For this review, take the finished solid that the model builds, in its own axes (mm). A direction names the side the tool comes from. Coordinates: 2 decimals unless noted, no trailing zeros. Write each loop counter-clockwise with the first axis right and the second up, starting at its lowest first coordinate (ties: lowest second). Pieces come first, ordered by that corner, then holes. Notation, with made-up numbers: (-31, 43) - (-5, 43) arc R16 cw to (-5, 56) - close; hole circle Ø1 at (43.5, -10). An arc over 180 degrees is marked (long way). Use one line per item in the form item = value. Start each with the question number.
1) We need section C-C (z = 0). Give the boundary of the cut face in (x, y), plus the area to 3 significant figures.
2) We need section B-B (y = 9.5). Give the boundary of the cut face in (x, z).
3) Mouldability with a two-part tool opening along Z and no side actions: class faces 3 (the flat face through (0, 0, 8)), 4 (the cylindrical face through (0.3, 11.6, -13.5)), 5 (the cylindrical face through (0.207, 11.661, 9.778)) as pulls with the +Z half, pulls with the -Z half, needs draft (parallel to the pull), parting line crosses it, or undercut.
4) Tool access review of faces 1 (the flat face through (0, 0.45, -15)), 2 (the cylindrical face through (0.3, 23.3, -3.6)): name each direction out of +Z, -Z, +X, -X, +Y, -Y from which nothing blocks a thin tool from reaching the whole face with its end or side.
5) Insertion check: P1, Ø1, axis at x = 0, z = -15.5, coming from the -Y side. The pin has a flat end and moves straight along its axis. Give the tip position at first contact, or say it passes through.
6) For L1, parallel to Z at x = -0.1, y = 21.5; L2, parallel to Y at x = -0.1, z = -7; L3, parallel to X at y = 25, z = 4, list the stretches that pass through material, from the lowest coordinate up. Write a range as from..to.
Autodesk Inventor part; units mm, degrees
ref_plane "YZ Plane" through (0, 0, 0) normal (1, 0, 0) x (0, 1, 0)
ref_plane "XZ Plane" through (0, 0, 0) normal (0, 1, 0) x (-1, 0, 0)
ref_plane "XY Plane" through (0, 0, 0) normal (0, 0, 1) x (1, 0, 0)
sketch "Boceto1" plane through (0, 0, 0) normal (1, 0, 0) x (0, 1, 0)
  line L0 (0, 8.3393) -> (23, 8.3393)
  line L1 (25, 6.3393) -> (25, -13.2007)
  line L2 (23, -15.2007) -> (0.45, -15.2007)
  arc A0 (25, 6.3393) -> (23, 8.3393) centre (23, 6.3393) ccw
  arc A1 (23, -15.2007) -> (25, -13.2007) centre (23, -13.2007) ccw
  line L3 (0, 13.6272) -> (0, -20.4886)
  point P0 (0, 0)
  point P1 (25, 8.3393)
  point P2 (25, -15.2007)
  dimension "d0" = 25
  dimension "d2" = 23.54
  dimension "d6" = 2
  dimension "d8" = 24.55
  dimension "d9" = 25
sketch "Boceto2" plane through (0, 0, 0) normal (0, 1, 0) x (-1, 0, 0)
  circle A0 centre (0, 8.2018) radius 1.59
  point P0 (0, 0)
  dimension "d3" = 3.18
sweep "Barrido1" add profiles "Boceto2" path "Boceto1" path curves L0 A0 L1 A1 L2
properties part number "BRAZOS BAILARINA"
Determined:
q1.outline = circle Ø3.18 at (0, 24.86)
q1.area = 7.94 mm²
q2.outline = circle Ø3.18 at (0, -15.06); circle Ø3.18 at (0, 8.2)
q3.face_3 = needs draft
q3.face_4 = undercut
q3.face_5 = undercut
q4.face_1 = -Z, +X, -X, -Y
q4.face_2 = none
q5.P1 = 0.45
q6.L1 = -16.65..-13.48, 6.61..9.79
q6.L2 = 23.28..26.45
q6.L3 = -1.58..1.58
